from build123d import *

# Parameters (mm, degrees)
IZIM1_R                     = 7.5
IZIM1_R_2                   = 1.5
Y_KSEKLIK_EKSTR_ZYON1_DEPTH = 10
KES_EKSTR_ZYON1_DEPTH       = 4
IZIM3_R                     = 11.025
KES_EKSTR_ZYON2_DEPTH       = 69


with BuildPart() as part:
    # Çizim1 → Yükseklik-Ekstrüzyon1 (new body)
    with BuildSketch(Plane.XY):
        with BuildLine():
            Line((-38.151258574, 18.853667601), (0, 10))
            Line((0, 10), (26.4, 10))
            Line((26.4, 10), (26.4, -10))
            Line((26.4, -10), (0, -10))
            Line((0, -10), (-38.151258574, -18.853667601))
            ThreePointArc((-38.151258574, -18.853667601), (-68.4, 0), (-38.151258574, 18.853667601))
        make_face()
        with Locations((-47.4, 0)):
            Circle(IZIM1_R, mode=Mode.SUBTRACT)
        with Locations((-16.4, 0)):
            Circle(IZIM1_R_2, mode=Mode.SUBTRACT)
        with Locations((-6.4, 0)):
            Circle(IZIM1_R_2, mode=Mode.SUBTRACT)
        with Locations((3.6, 0)):
            Circle(IZIM1_R_2, mode=Mode.SUBTRACT)
        with Locations((13.6, 0)):
            Circle(IZIM1_R_2, mode=Mode.SUBTRACT)
    extrude(amount=Y_KSEKLIK_EKSTR_ZYON1_DEPTH)

    # Çizim2 → Kes-Ekstrüzyon1 (cut)
    with BuildSketch(Plane.XY.offset(10)):
        Polygon((-25.98, -16.029113924), (0, -10), (26.4, -10), (26.4, 10), (0, 10), (-25.98, 16.029113924), align=None)
    extrude(amount=-KES_EKSTR_ZYON1_DEPTH, mode=Mode.SUBTRACT)

    # Çizim3 → Kes-Ekstrüzyon2 (cut)
    with BuildSketch(Plane.XY.offset(10)):
        with Locations((-47.4, 0)):
            Circle(IZIM3_R)
    extrude(amount=-KES_EKSTR_ZYON2_DEPTH, mode=Mode.SUBTRACT)


solid = part.part
Build history of the part. All positions in model axes, mm. A direction names the side the tool comes from. Round coordinates to 2 decimals unless told otherwise and drop trailing zeros. Loops run counter-clockwise (first coordinate to the right, second up) from the corner with the lowest first, then second, coordinate; pieces in that order, holes last. Notation, with made-up numbers: (71, -19.5) -> (128, -19.5) arc R24 ccw to (128, 6.5) -> close; hole circle Ø11 at (25.5, 57.5). An arc over 180 degrees is marked (long way). Answer in a Markdown table with one row per item.
Item 1: Mould opens along Y. For faces 1 (the cylindrical face through (-68.39, -0.6, 4.93)), 2 (the cylindrical face through (-36.884, 3.312, 5.07)), 3 (the flat face through (-20, 0, 0)), 4 (the flat face through (13, 10, 3)) say: +Y half, -Y half, draft (parallel to the pull), parting line (faces both ways), or undercut.
Answers below:
| item | result |
|---|---|
| face 1 | parting line |
| face 2 | undercut |
| face 3 | draft |
| face 4 | +Y half |
Item 2: Drill centre lines: L1, parallel to Y at x = 3.6, z = 3.15; L2, parallel to Z at x = 5, y = -7; L3, parallel to Y at x = 1, z = 2. Where is each one in solid material? Low to high. Write a range as [from, to].
Answers below:
| item | result |
|---|---|
| L1 | y = [-10, -1.5], [1.5, 10] |
| L2 | z = [0, 6] |
| L3 | y = [-10, 10] |
Item 3: Which spindle directions (+Z, -Z, +X, -X, +Y, -Y) get a long thin tool onto all of the face, cutting with end or side? Do faces 5 (the flat face through (13, -10, 3)), 6 (the flat face through (-25.98, 0, 8)), 7 (the cylindrical face through (-5.014, -0.575, 2.958)). Say none if no direction does.
Answers below:
| item | result |
|---|---|
| face 5 | +Z, -Z, +X, -Y |
| face 6 | +Z, +X, +Y, -Y |
| face 7 | +Z, -Z |
Item 4: Saw through at C-C (x = 3.6). Write the cut outline in (y, z).
Answers below:
| item | result |
|---|---|
| outline | (-10, 0) -> (-1.5, 0) -> (-1.5, 6) -> (-10, 6) -> close; (1.5, 0) -> (10, 0) -> (10, 6) -> (1.5, 6) -> close |
Item 5: Saw through at B-B (z = 3). Write the cut outline in (x, y) (3 decimals).
Answers below:
| item | result |
|---|---|
| outline | (-38.151, -18.854) -> (0, -10) -> (26.4, -10) -> (26.4, 10) -> (0, 10) -> (-38.151, 18.854) arc R21 ccw (long way) to start; hole circle Ø22.05 at (-47.4, 0); hole circle Ø3 at (-16.4, 0); hole circle Ø3 at (-6.4, 0); hole circle Ø3 at (3.6, 0); hole circle Ø3 at (13.6, 0) |
Item 6: Saw through at D-D (z = 7.5). Write the cut outline in (x, y) (3 decimals).
Answers below:
| item | result |
|---|---|
| outline | (-38.151, -18.854) -> (-25.98, -16.029) -> (-25.98, 16.029) -> (-38.151, 18.854) arc R21 ccw (long way) to start; hole circle Ø22.05 at (-47.4, 0) |
Item 7: Saw through at A-A (y = 0). Write the cut outline in (x, z) (3 decimals), and give its area (3 significant figures).
Answers below:
| item | result |
|---|---|
| outline | (-68.4, 0) -> (-58.425, 0) -> (-58.425, 10) -> (-68.4, 10) -> close; (-36.375, 0) -> (-17.9, 0) -> (-17.9, 6) -> (-25.98, 6) -> (-25.98, 10) -> (-36.375, 10) -> close; (-14.9, 0) -> (-7.9, 0) -> (-7.9, 6) -> (-14.9, 6) -> close; (-4.9, 0) -> (2.1, 0) -> (2.1, 6) -> (-4.9, 6) -> close; (5.1, 0) -> (12.1, 0) -> (12.1, 6) -> (5.1, 6) -> close; (15.1, 0) -> (26.4, 0) -> (26.4, 6) -> (15.1, 6) -> close |
| area | 446 mm² |
Item 8: Pin check, flat tips, straight feed: pin 1 (3 mm diameter, centred on y = 1, z = 8, fed in from +X); pin 2 (5 mm diameter, centred on y = -13, z = 7, fed in from -X); pin 3 (1.8 mm diameter, centred on x = 11.5, z = 4, fed in from -Y). Stop position of each tip, or through.
Answers below:
| item | result |
|---|---|
| pin 1 | stops at x = -25.98 |
| pin 2 | stops at x = -65.59 |
| pin 3 | stops at y = -10 |
